Geometry check sheet. Reference: the model listing, model coordinates, mm. A direction names the side the tool comes from. Coordinates: 2 decimals unless noted, no trailing zeros. Write each loop counter-clockwise with the first axis right and the second up, starting at its lowest first coordinate (ties: lowest second). Pieces come first, ordered by that corner, then holes. Notation, with made-up numbers: (42, -18) - (63, -18) arc R20 ccw to (63, 3) - close; hole circle Ø8 at (-28.5, -11). An arc over 180 degrees is marked (long way). Answer as a JSON object with one key per item and string values. Group by question number.
from build123d import *

# Parameters (mm, degrees)
SKETCH1_R           = 6.35
BOSS_EXTRUDE1_DEPTH = 278
BOSS_EXTRUDE2_START = -70.2975
SKETCH2_R           = 9.525
BOSS_EXTRUDE2_DEPTH = 146
CUT_EXTRUDE4_DEPTH  = 20


with BuildPart() as part:
    # Sketch1 → Boss-Extrude1 (new body)
    with BuildSketch(Plane.XY):
        Circle(SKETCH1_R)
    extrude(amount=BOSS_EXTRUDE1_DEPTH)

    # Sketch2 → Boss-Extrude2 (add)
    with BuildSketch(Plane(origin=(0, 0, 0), x_dir=(-1, 0, 0), z_dir=(0, 0, -1)).offset(BOSS_EXTRUDE2_START)):
        Circle(SKETCH2_R)
    extrude(amount=-BOSS_EXTRUDE2_DEPTH)

    # Sketch7 → Cut-Extrude4 (cut)
    with BuildSketch(Plane.XY):
        with BuildLine():
            Line((-5.499261314, 3.175), (5.499261314, 3.175))
            ThreePointArc((5.499261314, 3.175), (0, 6.35), (-5.499261314, 3.175))
        make_face()
    extrude(amount=CUT_EXTRUDE4_DEPTH, mode=Mode.SUBTRACT)


solid = part.part
(1) Set-up check for faces 1 (the face through (0, 3.175, 10)), 2 (the face through (-2, -6.2, 70.298)), 3 (the face through (0, 0, 278)), 4 (the face through (0, 0, 0)), 5 (the face through (-1.38, -6.2, 246.72)): record each of +Z, -Z, +X, -X, +Y, -Y from which the full face is reachable in a straight line by a thin tool's end or side.
(2) Section check D-D (z = 170). Record the cut outline in (x, y) (3 decimals), and give its area (3 significant figures).
(3) Gauge pin test, flat ends, axial feed: pin 1 (1 mm diameter, centred on x = 2, y = 5.5, fed in from -Z); pin 2 (3 mm diameter, centred on x = 5, z = 97, fed in from -Y); pin 3 (5 mm diameter, centred on x = -2, y = -5, fed in from -Z); pin 4 (6 mm diameter, centred on y = -2, z = 245, fed in from -X). Record the tip position at first contact, or that the pin passes through.
(4) Material ranges on L1, parallel to Z at x = 7.5, y = 4.75; L2, parallel to X at y = -0.5, z = 259; L3, parallel to X at y = -0.5, z = 171.5, recorded low to high. Write a range as [from, to].
(5) Section check C-C (z = 31). Record the cut outline in (x, y), and give its area (3 significant figures).
Conclusion:
{
 "1": {"face 1": "-Z, +X, -X, +Y", "face 2": "-Z", "face 3": "+Z, +X, -X, +Y, -Y", "face 4": "-Z, +X, -X, +Y, -Y", "face 5": "+Z"},
 "2": {"outline": "circle Ø19.05 at (0, 0)", "area": "285 mm^2"},
 "3": {"pin 1": "stops at z = 20", "pin 2": "stops at y = -8.86", "pin 3": "stops at z = 0", "pin 4": "stops at x = -6.35"},
 "4": {"L1": "z = [70.3, 216.3]", "L2": "x = [-6.33, 6.33]", "L3": "x = [-9.51, 9.51]"},
 "5": {"outline": "circle Ø12.7 at (0, 0)", "area": "127 mm^2"}
}
